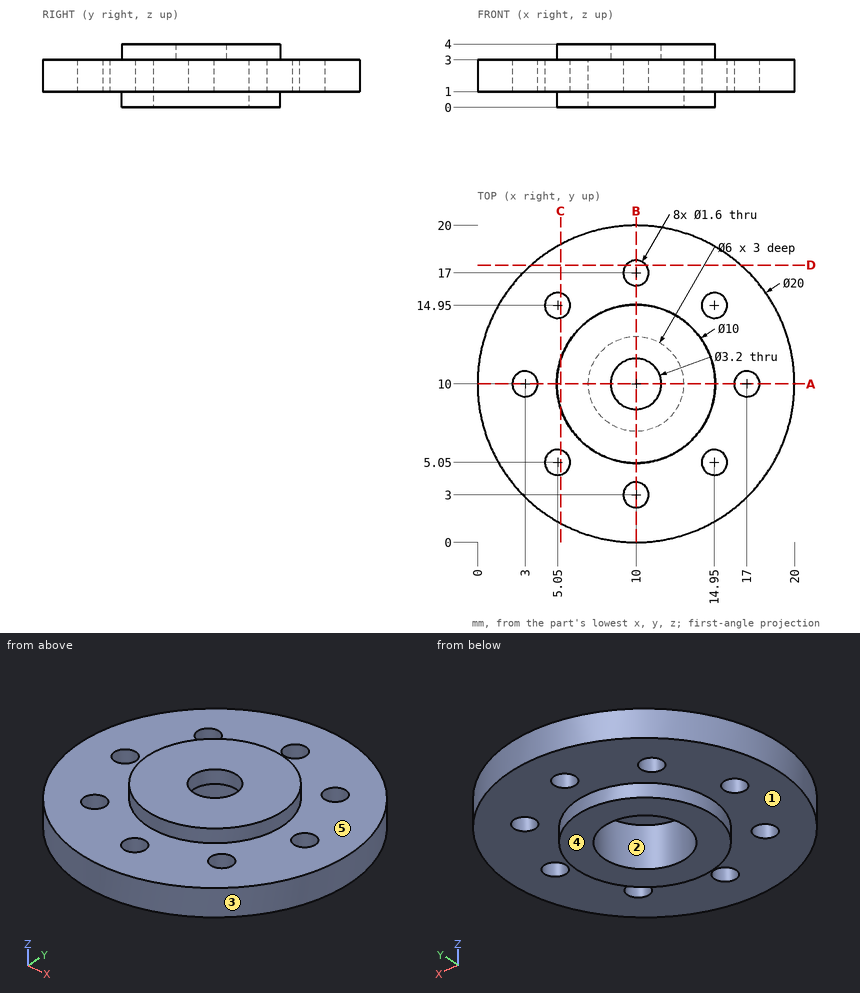
Source: three-view drawing plus pictorial views. Frame: mm from the lowest corner of the part. A direction names the side the tool comes from. Round coordinates to 2 decimals unless told otherwise and drop trailing zeros. Loops run counter-clockwise (first coordinate to the right, second up) from the corner with the lowest first, then second, coordinate; pieces in that order, holes last. Notation, with made-up numbers: M 14.5,-11.5 L 24.5,-11.5 A18 cw 24.5,14.5 Z; hole C 16,0.5 d7. An arc over 180 degrees is marked long. Put each result on its own line as item: value. Start each with the question number.
(1) Set-up query: the marked faces 4 and 5. Return all of +Z, -Z, +X, -X, +Y, -Y with unobstructed straight access to the full face (end or side cutting, diameter ignored); none if empty.
(2) Contact query for flat-ended pins moving along their axis: pin 1 Ø1 at (x, y) = (5.05, 14.95) entering from -Z (3 decimals); pin 2 Ø5 at (x, y) = (6.5, 3.5) entering from -Z; pin 3 Ø2 at (x, y) = (14.95, 5.05) entering from +Z; pin 4 Ø1 at (y, z) = (18, 3) entering from +X (1 decimal). Output: stop coordinate, or through.
(3) Section query C-C (x = 5.25). Return loops of the section in (y, z) (1 decimal).
(4) Section query A-A (y = 10). Return loops of the section in (x, z).
(5) Material intervals for line 1 along Y through (x, z) = (10, 2.2); line 2 along Y through (x, z) = (4.5, 1.1); line 3 along X through (y, z) = (14.75, 1.5) (1 decimal), sorted ascending. Write a range as [from, to].
(6) Draft query along Y for the marked faces 1, 2 and 3. Return one class per face: +Y half, -Y half, draft (parallel to the pull), parting line (faces both ways), or undercut.
(7) Section query D-D (y = 17.5). Return loops of the section in (x, z) (1 decimal).
Findings below:
1. face 4: -Z, +X, -X, +Y, -Y
1. face 5: +Z
2. pin 1: passes through
2. pin 2: stops at z = 0
2. pin 3: stops at z = 3
2. pin 4: stops at x = 16.6
3. outline: M 1.2,1 L 4.3,1 L 4.3,3 L 1.2,3 Z; M 5.8,1 L 8.4,1 L 8.4,0 L 11.6,0 L 11.6,1 L 14.2,1 L 14.2,3 L 11.6,3 L 11.6,4 L 8.4,4 L 8.4,3 L 5.8,3 Z; M 15.7,1 L 18.8,1 L 18.8,3 L 15.7,3 Z
4. outline: M 0,1 L 2.2,1 L 2.2,3 L 0,3 Z; M 3.8,1 L 5,1 L 5,0 L 7,0 L 7,3 L 8.4,3 L 8.4,4 L 5,4 L 5,3 L 3.8,3 Z; M 11.6,3 L 13,3 L 13,0 L 15,0 L 15,1 L 16.2,1 L 16.2,3 L 15,3 L 15,4 L 11.6,4 Z; M 17.8,1 L 20,1 L 20,3 L 17.8,3 Z
5. line 1: y = [0, 2.2], [3.8, 7], [13, 16.2], [17.8, 20]
5. line 2: y = [1.65, 4.47], [5.63, 14.37], [15.53, 18.35]
5. line 3: x = [1.2, 4.3], [5.8, 14.2], [15.7, 18.8]
6. face 1: draft
6. face 2: undercut
6. face 3: parting line
7. outline: M 3.4,1 L 9.4,1 L 9.4,3 L 3.4,3 Z; M 10.6,1 L 16.6,1 L 16.6,3 L 10.6,3 Z
